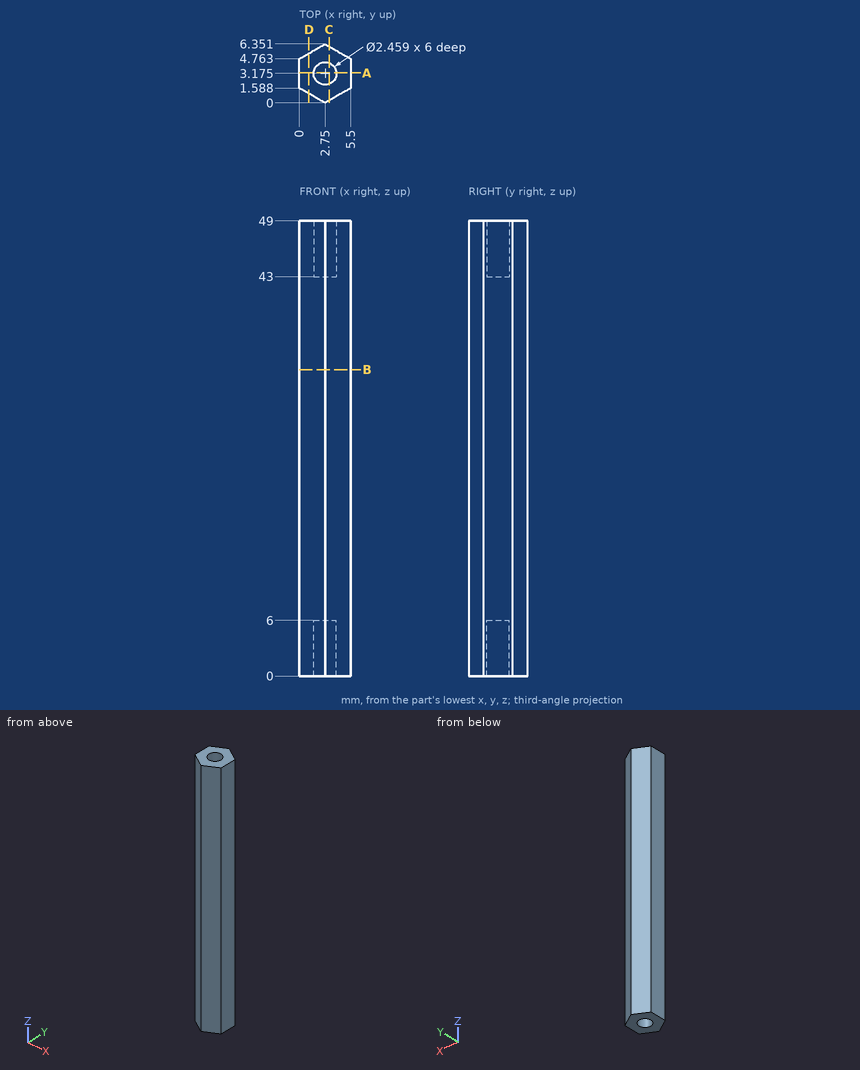
Drawing for the job (mm, zero at the part's lowest x, y, z). Give positions to 0.01 mm unless a question says otherwise; leave off trailing zeros. Order: outer loops, then holes, each group sorted by start corner. A loop starts at its lowest first (then second) coordinate and runs counter-clockwise, first axis right, second up. Notation, with made-up numbers: M 75,22.25 L 83,22.25 A10 cw 83,26.25 Z; hole C -5,-10 d4. An arc over 180 degrees is marked long. Put each result on its own line as item: value.
Item 1: Slice it at C-C, the plane x = 3.2. Write the cut outline in (y, z), plus the area to 3 significant figures.
From the geometry:
outline: M 0.26,0 L 2.03,0 L 2.03,6 L 4.32,6 L 4.32,0 L 6.09,0 L 6.09,49 L 4.32,49 L 4.32,43 L 2.03,43 L 2.03,49 L 0.26,49 Z
area: 258 mm2
Item 2: Slice it at D-D, the plane x = 1. Write the cut outline in (y, z), plus the area to 3 significant figures.
From the geometry:
outline: M 1.01,0 L 5.34,0 L 5.34,49 L 1.01,49 Z
area: 212 mm2
Item 3: Slice it at A-A, the plane y = 3.25. Write the cut outline in (x, z), plus the area to 3 significant figures.
From the geometry:
outline: M 0,0 L 1.52,0 L 1.52,6 L 3.98,6 L 3.98,0 L 5.5,0 L 5.5,49 L 3.98,49 L 3.98,43 L 1.52,43 L 1.52,49 L 0,49 Z
area: 240 mm2
Item 4: Probe line 1 (X direction, y = 2.25, z = 4.5); line 2 (Z direction, x = 2.7, y = 3); line 3 (X direction, y = 4, z = 47.5). List the from-to ranges inside material, lowest first. Write a range as [from, to].
From the geometry:
line 1: x = [0, 1.94], [3.56, 5.5]
line 2: z = [6, 43]
line 3: x = [0, 1.84], [3.66, 5.5]
Item 5: Slice it at B-B, the plane z = 33. Write the cut outline in (x, y), plus the area to 3 significant figures.
From the geometry:
outline: M 0,1.59 L 2.75,0 L 5.5,1.59 L 5.5,4.76 L 2.75,6.35 L 0,4.76 Z
area: 26.2 mm2
Item 6: Flat gauge pin, fed straight in: pin 1 Ø1.2 at (x, y) = (2.5, 3) entering from -Z. Where does the tip first touch, or does it go through?
From the geometry:
pin 1: stops at z = 6
